For this review, take the finished solid that the model builds, in its own axes (mm). Face numbers are marked on the shaded views. A direction names the side the tool comes from. Round coordinates to 2 decimals unless told otherwise and drop trailing zeros. Write each loop counter-clockwise with the first axis right and the second up, starting at its lowest first coordinate (ties: lowest second). Pieces come first, ordered by that corner, then holes. Notation, with made-up numbers: (-20, 30.25) - (-13, 30.25) arc R30 cw to (-13, 59.25) - close; hole circle Ø1 at (71.25, 2.5). An arc over 180 degrees is marked (long way). One line per item, written item: value. Start each with the question number.
Q1. For probe 1 along Z at (x, y) = (-0.05, 0.3); probe 2 along X at (y, z) = (0.4, -7.75); probe 3 along Z at (x, y) = (-1.3, 0.45), list the stretches that pass through material, from the lowest coordinate up.
Q2. Add section B-B on z = -6.25. Write out the cut boundary in (x, y).
Q3. Clearance check with a flat-ended pin moving along its axis: pin 1 Ø2 at (x, y) = (0.5, 0) entering from +Z. State where the tip first meets the part, or that it passes through.
Q4. Add section A-A on y = 0. Write out the cut boundary in (x, z), and give its area (3 significant figures).
Q5. Tool access review of the marked faces 1 and 2: name each direction out of +Z, -Z, +X, -X, +Y, -Y from which nothing blocks a thin tool from reaching the whole face with its end or side.
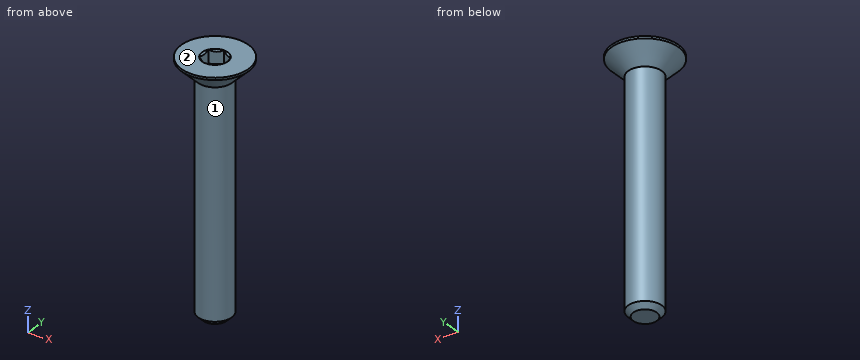
```python
from build123d import *

# Parameters (mm, degrees)
SKETCH3_W          = 22
SKETCH3_H          = 1.5
CHAMFER1_SIZE      = 0.45
CUT_EXTRUDE1_DEPTH = 1.19


with BuildPart() as part:
    # Sketch3 → Revolve1 (revolve)
    with BuildSketch(Plane(origin=(0, 0, 0), x_dir=(0, 0, -1), z_dir=(1, 0, 0))):
        with Locations((0, 0.75)):
            Rectangle(SKETCH3_W, SKETCH3_H)
    revolve(axis=Axis((0, 0, -11), (0, 0, 1)))

    # Chamfer1
    chamfer1_edges = [part.edges().sort_by_distance(p)[0] for p in [
        (0, -1.5, -11),
    ]]
    chamfer(chamfer1_edges, length=CHAMFER1_SIZE)

    # Sketch6 → Revolve2 (revolve)
    with BuildSketch(Plane(origin=(0, 0, 0), x_dir=(0, 0, -1), z_dir=(1, 0, 0))):
        Polygon((-11, 3), (-10.8, 3), (-9.3, 1.5), (-9.3, 0), (-11, 0), align=None)
    revolve(axis=Axis((0, 0, -11), (0, 0, 1)))

    # Sketch8 → Cut-Extrude1 (cut)
    with BuildSketch(Plane.XY.offset(11)):
        Polygon((0, 1.154700538), (-1, 0.577350269), (-1, -0.577350269), (0, -1.154700538), (1, -0.577350269), (1, 0.577350269), align=None)
    extrude(amount=-CUT_EXTRUDE1_DEPTH, mode=Mode.SUBTRACT)

    # Cut-Extrude2 cone 1 section (through the dimple's axis) → Cut-Extrude2 (revolve, cut)
    with BuildSketch(Plane(origin=(0, 0, 11), x_dir=(0, -1, 0), z_dir=(1, 0, 0))):
        Polygon((0, 0), (1.154700538, 0), (0, 1.154700538), align=None)
    revolve(axis=Axis((0, 0, 11), (0, 0, -1)), mode=Mode.SUBTRACT)


solid = part.part
```
Result set:
1. probe 1: z = -11 to 9.81
1. probe 2: x = -1.45 to 1.45
1. probe 3: z = -10.67 to 11
2. outline: circle Ø3 at (0, 0)
3. pin 1: stops at z = 11
4. outline: (-3, 10.8) - (-1.5, 9.3) - (-1.5, -10.55) - (-1.05, -11) - (1.05, -11) - (1.5, -10.55) - (1.5, 9.3) - (3, 10.8) - (3, 11) - (1.15, 11) - (1, 10.85) - (1, 9.81) - (-1, 9.81) - (-1, 10.85) - (-1.15, 11) - (-3, 11) - close
4. area: 66.2 mm^2
5. face 1: -Z
5. face 2: +Z, +X, -X, +Y, -Y
